```python
from build123d import *

# Parameters (mm, degrees)
F0_R     = 9.525
F0_R_2   = 7.9375
F1_DEPTH = 38.1
F2_W     = 19.05
F2_H     = 3.175
F3_DEPTH = 44.45
F4_R     = 5.08
F5_R     = 7.9375
F6_DEPTH = 114.3


with BuildPart() as f1:
    # F0 (on Top) → F1 (new body, symmetric)
    with BuildSketch(Plane.XY):
        Circle(F0_R)
        Circle(F0_R_2, mode=Mode.SUBTRACT)
    extrude(amount=F1_DEPTH, both=True)

    # F2 (on Right) → F3 (join)
    with BuildSketch(Plane.YZ):
        Rectangle(F2_W, F2_H)
    extrude(amount=F3_DEPTH)

    # F4
    f4_edges = [f1.edges().sort_by_distance(p)[0] for p in [
        (44.45, -9.525, 0),
        (44.45, 9.525, 0),
    ]]
    fillet(f4_edges, radius=F4_R)

    # F5 (on Front) → F6 (join)
    with BuildSketch(Plane.XZ):
        Circle(F5_R)
    extrude(amount=F6_DEPTH)


solid = f1.part
```
The listing builds one solid part. Answer for the finished solid, in the listing's coordinates (mm). A direction names the side the tool comes from. Give positions to 0.01 mm unless a question says otherwise; leave off trailing zeros. Order: outer loops, then holes, each group sorted by start corner. A loop starts at its lowest first (then second) coordinate and runs counter-clockwise, first axis right, second up. Notation, with made-up numbers: (40, 60.25) - (86, 60.25) arc R29 ccw to (86, 89.25) - close; hole circle Ø8 at (49.5, 3). An arc over 180 degrees is marked (long way). Use one line per item in the form item = value. Start each with the question number.
(1) A cutting plane is placed at D-D, the plane x = 34. Write down the section's boundary in (y, z) (1 decimal), then the cut area to 3 significant figures.
(2) The mould has two halves that part along Y. Classify faces 1 (the flat face through (0, -114.3, 0)), 2 (the cylindrical face through (-0.64, -3.03, 7.91)), 3 (the cylindrical face through (-7.02, 6.44, 0.53)): released by +Y, released by -Y, zero draft, split by the parting line, or undercut.
(3) A cutting plane is placed at B-B, the plane x = -2.5. Write down the section's boundary in (y, z), then the cut area to 3 significant figures.
(4) Flat-ended cylindrical pins translate along their axes: pin 1 Ø5 at (x, y) = (8.5, -77.5) entering from -Z; pin 2 Ø1.6 at (y, z) = (2.5, 0.5) entering from -X; pin 3 Ø10 at (x, z) = (9, -11) entering from -Y. Find the tip coordinate at first contact, or state that the pin passes through.
(5) A cutting plane is placed at C-C, the plane y = -20.5. Write down the section's boundary in (x, z) (1 decimal), then the cut area to 3 significant figures.
(6) Consider line 1 (Y direction, x = 0, z = -20.5) (1 decimal); line 2 (Y direction, x = 0, z = 6) (1 decimal); line 3 (X direction, y = -2, z = -5). Determine where each line is inside the solid, lowest interval first. Write a range as from..to.
(7) For faces 4 (the flat face through (0, 4, 0)), 5 (the flat face through (3, 3, 1.588)), 6 (the flat face through (3, 3, -1.588)), determine the directions among +Z, -Z, +X, -X, +Y, -Y from which every point of the face is accessible in a straight line to the end or side of a thin tool.
Ans:
q1.outline = (-9.5, -1.6) - (9.5, -1.6) - (9.5, 1.6) - (-9.5, 1.6) - close
q1.area = 60.5 mm^2
q2.face_1 = released by -Y
q2.face_2 = undercut
q2.face_3 = split by the parting line
q3.outline = (-114.3, -7.53) - (-9.19, -7.53) - (-9.19, -38.1) - (-7.53, -38.1) - (-7.53, -7.53) - (0, -7.53) - (0, 7.53) - (-7.53, 7.53) - (-7.53, 38.1) - (-9.19, 38.1) - (-9.19, 7.53) - (-114.3, 7.53) - close; (7.53, -38.1) - (9.19, -38.1) - (9.19, 38.1) - (7.53, 38.1) - close
q3.area = 1,950 mm^2
q4.pin_1 = -5.2
q4.pin_2 = -9.37
q4.pin_3 = -8.64
q5.outline = circle Ø15.9 at (0, 0)
q5.area = 198 mm^2
q6.line_1 = -9.5..-7.9, 7.9..9.5
q6.line_2 = -114.3..0, 7.9..9.5
q6.line_3 = -9.31..-7.68, -6.16..6.16, 7.68..9.31
q7.face_4 = +Z, -Z
q7.face_5 = +Z
q7.face_6 = -Z
